```python
from build123d import *

# Parameters (mm, degrees)
SKETCH1_W           = 10
SKETCH1_H           = 45
BOSS_EXTRUDE1_DEPTH = 2
SKETCH2_R           = 3.5
CUT_EXTRUDE1_DEPTH  = 2
SKETCH3_R           = 3
BOSS_EXTRUDE2_DEPTH = 10


with BuildPart() as part:
    # Sketch1 → Boss-Extrude1 (new body)
    with BuildSketch(Plane(origin=(0, 0, 0), x_dir=(0, 0, -1), z_dir=(1, 0, 0))):
        Rectangle(SKETCH1_W, SKETCH1_H)
    extrude(amount=BOSS_EXTRUDE1_DEPTH)

    # Sketch2 → Cut-Extrude1 (cut)
    with BuildSketch(Plane(origin=(2, 0, 0), x_dir=(0, 0, -1), z_dir=(1, 0, 0))):
        with Locations((0, -16)):
            Circle(SKETCH2_R)
    extrude(amount=-CUT_EXTRUDE1_DEPTH, mode=Mode.SUBTRACT)

    # Sketch3 → Boss-Extrude2 (add)
    with BuildSketch(Plane(origin=(2, 0, 0), x_dir=(0, 0, -1), z_dir=(1, 0, 0))):
        with Locations((0, 16)):
            Circle(SKETCH3_R)
    extrude(amount=BOSS_EXTRUDE2_DEPTH)


solid = part.part
```
The model under review builds one solid part; all positions refer to its coordinate system, in mm. Coordinates: 2 decimals unless noted, no trailing zeros. Order: outer loops, then holes, each group sorted by start corner. A loop starts at its lowest first (then second) coordinate and runs counter-clockwise, first axis right, second up. Notation, with made-up numbers: M 55.5,22 L 60.5,22 A24 ccw 60.5,48 Z; hole C 33.25,-33 d8. An arc over 180 degrees is marked long. One line per question, with ' | ' between items.
(1) Insertion check: pin 1 (4 mm diameter, centred on x = 7.5, z = -1, fed in from -Y); pin 2 (4 mm diameter, centred on x = 4.5, y = -15, fed in from -Z); pin 3 (3 mm diameter, centred on x = 10, z = 3, fed in from +Y); pin 4 (6 mm diameter, centred on x = 8.5, y = 16.5, fed in from -Z). Each pin has a flat end and moves straight along its axis. Give the tip position at first contact, or say it passes through.
Geometry results:
pin 1: stops at y = 13 | pin 2: passes through | pin 3: stops at y = 18.6 | pin 4: stops at z = -3
(2) Add section A-A, the plane z = 0. Write out the cut boundary in (x, y), then the cut area to 3 significant figures.
Geometry results:
outline: M 0,-22.5 L 2,-22.5 L 2,-19.5 L 0,-19.5 Z; M 0,-12.5 L 2,-12.5 L 2,13 L 12,13 L 12,19 L 2,19 L 2,22.5 L 0,22.5 Z | area: 136 mm²
(3) Add section C-C, the plane y = 16. Write out the cut boundary in (x, z), then the cut area to 3 significant figures.
Geometry results:
outline: M 0,-5 L 2,-5 L 2,-3 L 12,-3 L 12,3 L 2,3 L 2,5 L 0,5 Z | area: 80.0 mm²
(4) Add section B-B, the plane y = -16. Write out the cut boundary in (x, z), then the cut area to 3 significant figures.
Geometry results:
outline: M 0,-5 L 2,-5 L 2,-3.5 L 0,-3.5 Z; M 0,3.5 L 2,3.5 L 2,5 L 0,5 Z | area: 6.00 mm²
(5) For probe 1 along Y at (x, z) = (0.6, 0); probe 2 along X at (y, z) = (4, 1.25); probe 3 along Y at (x, z) = (2.5, 0), list the stretches that pass through material, from the lowest coordinate up. Write a range as from..to.
Geometry results:
probe 1: y = -22.5..-19.5, -12.5..22.5 | probe 2: x = 0..2 | probe 3: y = 13..19
(6) The part is to be moulded in two halves that separate along Y. For faces 1 (the face through (1.014, -17.341, -3.233)), 2 (the face through (1, 22.5, 0)), 3 (the face through (6.93, 13.07, 0.65)), say which applies: +Y half, -Y half, draft (parallel to the pull), parting line (faces both ways), or undercut.
Geometry results:
face 1: undercut | face 2: +Y half | face 3: parting line
(7) Add section D-D, the plane x = 3. Write out the cut boundary in (y, z), then the cut area to 3 significant figures.
Geometry results:
outline: C 16,0 d6 | area: 28.3 mm²
